Here's how the part is built. I have some questions about the finished solid (model axes, mm). Face numbers are marked on the shaded views. A direction names the side the tool comes from. Round coordinates to 2 decimals unless told otherwise and drop trailing zeros. Order: outer loops, then holes, each group sorted by start corner. A loop starts at its lowest first (then second) coordinate and runs counter-clockwise, first axis right, second up. Notation, with made-up numbers: (85, 65) -> (119, 65) arc R20 cw to (119, 81) -> close; hole circle Ø7 at (65.5, 59.25). An arc over 180 degrees is marked (long way). Answer in a Markdown table with one row per item.
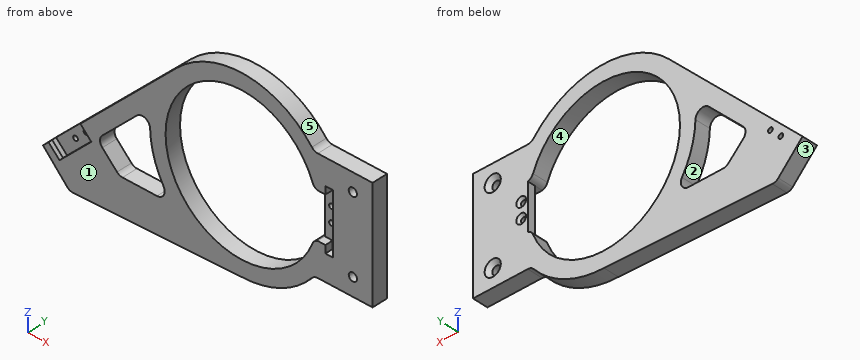
```python
from build123d import *

# Parameters (mm, degrees)
BOSS_EXTRUDE1_DEPTH                             = 5
FILLET1_R                                       = 5
CUT_EXTRUDE1_DEPTH                              = 10
F_3_0MM_PRESS_DOWEL_HOLE2_D                     = 3
F_3_0MM_PRESS_DOWEL_HOLE2_CSINK_D               = 3.05
F_3_0MM_PRESS_DOWEL_HOLE2_CSINK_ANGLE           = 90
CUT_EXTRUDE2_DEPTH                              = 5
CSK_FOR_M3_FLAT_HEAD_MACHINE_SCREW2_D           = 3.2
CSK_FOR_M3_FLAT_HEAD_MACHINE_SCREW2_CSINK_D     = 6.3
CSK_FOR_M3_FLAT_HEAD_MACHINE_SCREW2_CSINK_ANGLE = 90


with BuildPart() as part:
    # Sketch1 → Boss-Extrude1 (new, symmetric)
    with BuildSketch(Plane(origin=(0, 0, 0), x_dir=(1, 0, 0), z_dir=(0, 1, 0))):
        with BuildLine():
            Line((-107.462553071, 24.023952891), (-41.71930009, -41.71930009))
            ThreePointArc((-41.71930009, -41.71930009), (3.806502253, -58.877079926), (46.74398357, -36))
            Line((46.74398357, -36), (84.4, -36))
            Line((84.4, -36), (84.4, 36))
            Line((84.4, 36), (46.74398357, 36))
            ThreePointArc((46.74398357, 36), (26.048032555, 52.93864373), (0, 59))
            Line((0, 59), (-110.83863918, 62.740943777))
            Line((-110.83863918, 62.740943777), (-128.004005064, 44.565404884))
            Line((-128.004005064, 44.565404884), (-107.462553071, 24.023952891))
        make_face()
        with BuildLine():
            Line((49, 14.576290822), (46.781745862, 14.576290822))
            ThreePointArc((46.781745862, 14.576290822), (-49, 0), (46.781745862, -14.576290822))
            Line((46.781745862, -14.576290822), (49, -14.576290822))
            Line((49, -14.576290822), (49, 14.576290822))
        make_face(mode=Mode.SUBTRACT)
        with BuildLine():
            Line((-93.296148974, 23.999684418), (-57.886132355, -11.410332201))
            ThreePointArc((-57.886132355, -11.410332201), (-57.048958802, 15.047135926), (-44.728269399, 38.475731527))
            Line((-44.728269399, 38.475731527), (-78.820101865, 38.475731527))
            Line((-78.820101865, 38.475731527), (-93.296148974, 23.999684418))
        make_face(mode=Mode.SUBTRACT)
    extrude(amount=BOSS_EXTRUDE1_DEPTH, both=True)

    # Fillet1
    # the kernel refuses this fillet: 5 mm, written as the material it adds along each edge
    with BuildSketch(Plane(origin=(46.74398357, -5, 36), x_dir=(1, 0, 0), z_dir=(0, 1, 0))) as fillet1_piece_1:
        with BuildLine():
            CenterArc((2.398665931, -5), FILLET1_R, 90, 50.161560023)
            ThreePointArc((-1.440603561, -1.796875), (-0.711533327, -0.905467408), (0, 0))
            Line((0, 0), (2.398665931, 0))
        make_face()
    extrude(amount=10)
    with BuildSketch(Plane(origin=(46.74398357, -5, -36), x_dir=(-0.6255163967442842, 0, -0.7802110210731757), z_dir=(0, 1, 0))) as fillet1_piece_2:
        with BuildLine():
            CenterArc((2.400650235, -4.999047579), FILLET1_R, 91.118340331, 50.161560023)
            Line((-1.50040487, -1.871465595), (0, 0))
            ThreePointArc((0, 0), (1.151531414, -0.011238567), (2.303062827, 0))
        make_face()
    extrude(amount=10)
    with BuildSketch(Plane(origin=(-93.296148974, -5, -23.999684418), x_dir=(0.7071067811865472, 0, -0.7071067811865479), z_dir=(0, 1, 0))) as fillet1_piece_3:
        with BuildLine():
            CenterArc((FILLET1_R, -FILLET1_R), FILLET1_R, 90, 90)
            Line((0, -FILLET1_R), (0, 0))
            Line((0, 0), (FILLET1_R, 0))
        make_face()
    extrude(amount=10)
    with BuildSketch(Plane(origin=(-78.820101865, -5, -38.475731527), x_dir=(1, 0, 0), z_dir=(0, 1, 0))) as fillet1_piece_4:
        with BuildLine():
            CenterArc((FILLET1_R * 0.414213562373, -FILLET1_R), FILLET1_R, 90, 45)
            Line((-FILLET1_R * 0.292893218813, -FILLET1_R * 0.292893218813), (0, 0))
            Line((0, 0), (FILLET1_R * 0.414213562373, 0))
        make_face()
    extrude(amount=10)
    with BuildSketch(Plane(origin=(-57.886132355, -5, 11.410332201), x_dir=(-0.7071067811865467, 0, -0.7071067811865482), z_dir=(0, 1, 0))) as fillet1_piece_5:
        with BuildLine():
            CenterArc((13.612446704, -5), FILLET1_R, 90, 133.432536558)
            ThreePointArc((9.981524817, -8.4375), (5.225121697, -3.941504009), (0, 0))
            Line((0, 0), (13.612446704, 0))
        make_face()
    extrude(amount=10)
    with BuildSketch(Plane(origin=(-44.728269399, 5, -38.475731527), x_dir=(-1, 0, 0), z_dir=(0, -1, 0))) as fillet1_piece_6:
        with BuildLine():
            CenterArc((9.81873234, -5), FILLET1_R, 90, 121.53762105)
            ThreePointArc((5.557247829, -7.615291526), (2.930969774, -3.696471595), (0, 0))
            Line((0, 0), (9.81873234, 0))
        make_face()
    extrude(amount=10)
    # the kernel refuses this fillet: 5 mm, written as the material it takes off along each edge
    with BuildSketch(Plane(origin=(46.781745862, 12.95259813, 14.576290822), x_dir=(-0.32830869078175484, 0, 0.9445704862831413), z_dir=(0, -1, 0)), Plane(origin=(46.781745862, -12.95259813, -14.576290822), x_dir=(-0.32830869078175745, 0, -0.9445704862831404), z_dir=(0, 1, 0))) as fillet1_2_piece_1:
        with BuildLine():
            CenterArc((3.343337173, -4.997365244), FILLET1_R, 91.860123923, 52.660239811)
            Line((-0.728272112, -2.09529739), (0, 0))
            ThreePointArc((0, 0), (1.590519626, -0.025820606), (3.181039252, 0))
        make_face()
    extrude(amount=25.90519626, mode=Mode.SUBTRACT)
    with BuildSketch(Plane(origin=(-110.83863918, 10.640073082, -62.740943777), x_dir=(-0.6866146353868613, 0, 0.7270215557138366), z_dir=(0, -1, 0))) as fillet1_2_piece_2:
        with BuildLine():
            CenterArc((FILLET1_R * 0.451205846565, -FILLET1_R), FILLET1_R, 90, 48.570349235)
            Line((-FILLET1_R * 0.298562891452, -FILLET1_R * 0.338300038165), (0, 0))
            Line((0, 0), (FILLET1_R * 0.451205846565, 0))
        make_face()
    extrude(amount=21.280146164, mode=Mode.SUBTRACT)

    # Sketch11 → Cut-Extrude1 (cut)
    with BuildSketch(Plane(origin=(-41.71930009, 0, 41.71930009), x_dir=(0.7071067811865458, 0, 0.7071067811865492), z_dir=(-0.7071067811865492, 0, 0.7071067811865458))):
        Polygon((-116.982839598, -5), (-116.982839598, -2.5), (-119.982839598, -2.5), (-119.982839598, 2.5), (-84.982839598, 2.5), (-84.982839598, -2.5), (-87.982839598, -2.5), (-87.982839598, -5), align=None)
    extrude(amount=-CUT_EXTRUDE1_DEPTH, mode=Mode.SUBTRACT)

    # Ø3.0mm Press Dowel Hole2 (through all)
    with Locations(Plane(origin=(-114.00883423, 5, -37.641301862), x_dir=(0, 0, 1), z_dir=(0, 1, 0))):
        with Locations((0, 0), (6.717514422, 6.717514421)):
            CounterSinkHole(F_3_0MM_PRESS_DOWEL_HOLE2_D / 2, F_3_0MM_PRESS_DOWEL_HOLE2_CSINK_D / 2, counter_sink_angle=F_3_0MM_PRESS_DOWEL_HOLE2_CSINK_ANGLE)

    # Sketch15 → Cut-Extrude2 (cut)
    with BuildSketch(Plane(origin=(0, -5, 0), x_dir=(-1, 0, 0), z_dir=(0, -1, 0))):
        Polygon((-49, -14.576290822), (-54, -14.576290822), (-54, -19.5), (-59, -19.5), (-59, 19.5), (-54, 19.5), (-54, 14.576290822), (-49, 14.576290822), align=None)
    extrude(amount=-CUT_EXTRUDE2_DEPTH, mode=Mode.SUBTRACT)

    # CSK for M3 Flat Head Machine Screw2 (through all)
    with Locations(Plane(origin=(53.32762779, 5, -4.850211012), x_dir=(0, 0, 1), z_dir=(0, 1, 0))):
        with Locations((0, 0), (9.700422024, 0)):
            CounterSinkHole(CSK_FOR_M3_FLAT_HEAD_MACHINE_SCREW2_D / 2, CSK_FOR_M3_FLAT_HEAD_MACHINE_SCREW2_CSINK_D / 2, counter_sink_angle=CSK_FOR_M3_FLAT_HEAD_MACHINE_SCREW2_CSINK_ANGLE)

    # CSK for M5 Flat Head Machine Screw2: read off the stored shape, not the designer's step
    # CSK for M5 Flat Head Machine Screw2 outl → CSK for M5 Flat Head Machine Screw2 (revolve, cut)
    with BuildSketch(Plane(origin=(71.691354027, 0, 24.5), x_dir=(1, 0, 0), z_dir=(0, 0, 1))):
        Polygon((0, -5), (2.65, -5), (2.65, 2.45), (5.2, 5), (0, 5), align=None)
    revolve(axis=Axis((71.691354027, 0, 24.5), (0, 1, 0)), mode=Mode.SUBTRACT)

    # CSK for M5 Flat Head Machine Screw2 2 ou → CSK for M5 Flat Head Machine Screw2 2 (revolve, cut)
    with BuildSketch(Plane(origin=(71.691354027, 0, -24.5), x_dir=(1, 0, 0), z_dir=(0, 0, 1))):
        Polygon((0, -5), (2.65, -5), (2.65, 2.45), (5.2, 5), (0, 5), align=None)
    revolve(axis=Axis((71.691354027, 0, -24.5), (0, 1, 0)), mode=Mode.SUBTRACT)


solid = part.part
```
1. Suppose I cut it at A-A on x = 14. Write out the boundary of the cut face in (y, z), then the cut area to 3 significant figures.
Numbers:
| item | result |
|---|---|
| outline | (-5, -57.31) -> (5, -57.31) -> (5, -46.96) -> (-5, -46.96) -> close; (-5, 46.96) -> (5, 46.96) -> (5, 57.31) -> (-5, 57.31) -> close |
| area | 207 mm2 |
2. Suppose I cut it at B-B on z = 24.5. Write out the boundary of the cut face in (x, y), then the cut area to 3 significant figures.
Numbers:
| item | result |
|---|---|
| outline | (-58.94, -5) -> (-42.44, -5) -> (-42.44, 5) -> (-58.94, 5) -> close; (42.44, -5) -> (69.04, -5) -> (69.04, 2.45) -> (66.49, 5) -> (42.44, 5) -> close; (74.34, -5) -> (84.4, -5) -> (84.4, 5) -> (76.89, 5) -> (74.34, 2.45) -> close |
| area | 525 mm2 |
3. We'd pull the mould along Z, two halves only. Please class the marked faces 3, 4 and 5: released by +Z, released by -Z, zero draft, split by the parting line, or undercut.
Numbers:
| item | result |
|---|---|
| face 3 | released by -Z |
| face 4 | undercut |
| face 5 | released by +Z |
4. Suppose I cut it at D-D on x = 37. Write out the boundary of the cut face in (y, z).
Numbers:
| item | result |
|---|---|
| outline | (-5, -45.96) -> (5, -45.96) -> (5, -32.12) -> (-5, -32.12) -> close; (-5, 32.12) -> (5, 32.12) -> (5, 45.96) -> (-5, 45.96) -> close |
5. For pin 1 Ø4 at (x, z) = (71.69, -24.5) entering from -Y; pin 2 Ø5 at (x, z) = (-114.01, -37.64) entering from +Y; pin 3 Ø5 at (y, z) = (-3.5, -47.5) entering from +X; pin 4 Ø4 at (x, y) = (56.5, -2) entering from -Z, each with a flat end and sliding along its axis, tell me the tip position at first contact or that it passes through.
Numbers:
| item | result |
|---|---|
| pin 1 | passes through |
| pin 2 | stops at y = 5 |
| pin 3 | stops at x = 38.16 |
| pin 4 | stops at z = -36 |
6. Suppose I cut it at C-C on z = 12. Write out the boundary of the cut face in (x, y), then the cut area to 3 significant figures.
Numbers:
| item | result |
|---|---|
| outline | (-71.44, -5) -> (-47.51, -5) -> (-47.51, 5) -> (-71.44, 5) -> close; (49, 0) -> (59, 0) -> (59, -5) -> (84.4, -5) -> (84.4, 5) -> (49, 5) -> close |
| area | 543 mm2 |
7. Please list where these lines run through material, in increasing order: line 1 along X through (y, z) = (-2.75, -35.5) (3 decimals); line 2 along X through (y, z) = (2, -10); line 3 along Z through (x, y) = (52.5, -1.5).
Numbers:
| item | result |
|---|---|
| line 1 | x = -104.796 to -81.796, -49.975 to -33.775, 33.775 to 84.4 |
| line 2 | x = -93.44 to -79.3, -58.15 to -47.97, 49 to 84.4 |
| line 3 | z = -36 to -14.58, 14.58 to 36 |
8. For the marked faces 1 and 2, which set-ups out of +Z, -Z, +X, -X, +Y, -Y let a thin tool reach every point of the face, with its end or its side?
Numbers:
| item | result |
|---|---|
| face 1 | +Z, -Z, +X, -X, -Y |
| face 2 | +Y, -Y |
